The drawing under review shows one solid part. Ordinate dimensions are in mm from its lowest x, y, z. Round coordinates to 2 decimals unless told otherwise and drop trailing zeros. Order: outer loops, then holes, each group sorted by start corner. A loop starts at its lowest first (then second) coordinate and runs counter-clockwise, first axis right, second up. Notation, with made-up numbers: (-12.5, -23) -> (-0.5, -23) arc R25 ccw to (-0.5, 6) -> close; hole circle Ø4 at (86, 72). An arc over 180 degrees is marked (long way). Use a Markdown table: item, result. Add a question column.
1) Consider section C-C (x = 74). State the section outline as (y, z) points, plus the area to 3 significant figures.
2) Consider section A-A (y = 20). State the section outline as (x, z) points.
3) Consider section B-B (z = 0.45). State the section outline as (x, y) points.
4) Wall thickness on line 1 along X through (y, z) = (21.25, 2.6); line 2 along Y through (x, z) = (83, 0.35): over which ranges is each line inside the solid? List them lowest first. Write a range as [from, to].
5) Clearance check with a flat-ended pin moving along its axis: P1, Ø0.9, axis at x = 94.5, z = 1.5, coming from the +Y side. State where the tip first meets the part, or that it passes through.
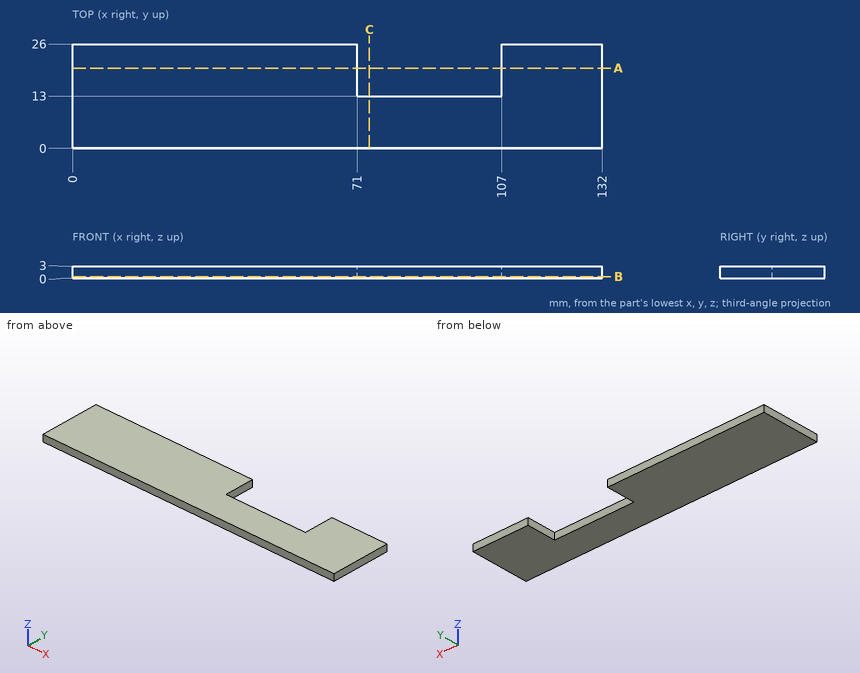
Results list:
| question | item | result |
|---|---|---|
| 1 | outline | (0, 0) -> (13, 0) -> (13, 3) -> (0, 3) -> close |
| 1 | area | 39.0 mm2 |
| 2 | outline | (0, 0) -> (71, 0) -> (71, 3) -> (0, 3) -> close; (107, 0) -> (132, 0) -> (132, 3) -> (107, 3) -> close |
| 3 | outline | (0, 0) -> (132, 0) -> (132, 26) -> (107, 26) -> (107, 13) -> (71, 13) -> (71, 26) -> (0, 26) -> close |
| 4 | line 1 | [0, 71], [107, 132] |
| 4 | line 2 | [0, 13] |
| 5 | P1 | y = 13 |
